Design review of the part shown in the three views and the two pictorial views. Dimensions are in mm from the part's minimum x, y and z. A direction names the side the tool comes from. Round coordinates to 2 decimals unless told otherwise and drop trailing zeros. Loops run counter-clockwise (first coordinate to the right, second up) from the corner with the lowest first, then second, coordinate; pieces in that order, holes last.
1) Insertion check: pin 1 (5.5 mm diameter, centred on x = 8.5, z = 9, fed in from -Y); pin 2 (1.5 mm diameter, centred on x = 10.5, z = 9.5, fed in from -Y); pin 3 (1.5 mm diameter, centred on y = 7, z = 13, fed in from -X); pin 4 (4.5 mm diameter, centred on x = 9.455, z = 9.455, fed in from +Y). Each pin has a flat end and moves straight along its axis. Give the tip position at first contact, or say it passes through.
2) Tool access review of the marked faces 1, 2 and 3: name each direction out of +Z, -Z, +X, -X, +Y, -Y from which nothing blocks a thin tool from reaching the whole face with its end or side.
3) Take a section at B-B (x = 11.5). State the section outline as (y, z) points.
4) Take a section at D-D (y = 9). State the section outline as (x, z) points (3 decimals), then the cut area to 3 significant figures.
5) Take a section at C-C (y = 2). State the section outline as (x, z) points (3 decimals).
6) Take a section at A-A (z = 9.25). State the section outline as (x, y) points.
7) Wall thickness on L1, parallel to Z at x = 8.25, y = 18.25; L2, parallel to X at y = 2.5, z = 10.75; L3, parallel to Z at x = 1.25, y = 15.25: over which ranges is each line inside the solid? List them lowest first.
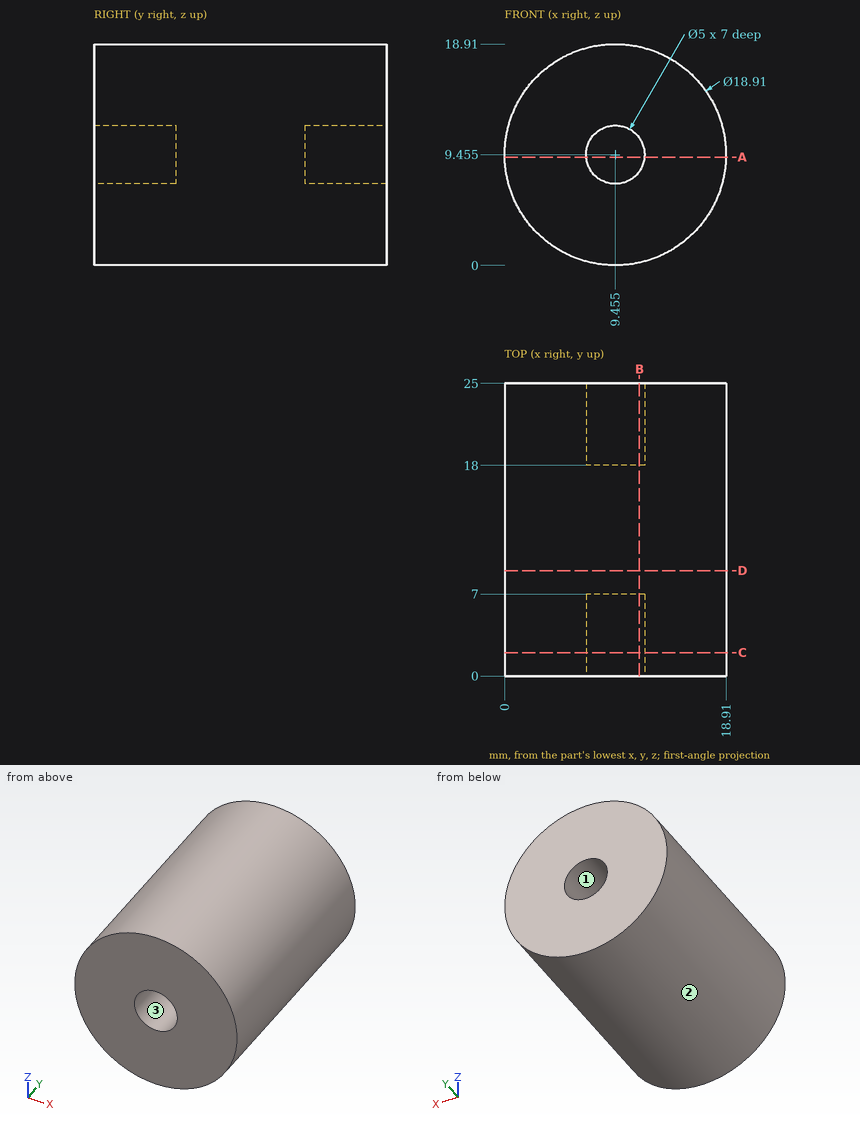
Response:
1. pin 1: stops at y = 0
1. pin 2: stops at y = 7
1. pin 3: stops at x = 0.42
1. pin 4: stops at y = 18
2. face 1: +Y
2. face 2: +Y, -Y
2. face 3: -Y
3. outline: (0, 0.22) - (25, 0.22) - (25, 8.02) - (18, 8.02) - (18, 10.89) - (25, 10.89) - (25, 18.69) - (0, 18.69) - (0, 10.89) - (7, 10.89) - (7, 8.02) - (0, 8.02) - close
4. outline: circle Ø18.91 at (9.455, 9.455)
4. area: 281 mm2
5. outline: circle Ø18.91 at (9.455, 9.455); hole circle Ø5 at (9.455, 9.455)
6. outline: (0, 0) - (6.96, 0) - (6.96, 7) - (11.95, 7) - (11.95, 0) - (18.91, 0) - (18.91, 25) - (11.95, 25) - (11.95, 18) - (6.96, 18) - (6.96, 25) - (0, 25) - close
7. L1: z = 0.08 to 7.26, 11.65 to 18.83
7. L2: x = 0.09 to 7.32, 11.59 to 18.82
7. L3: z = 4.76 to 14.15
